Part print with two shaded views. Sizes in mm from the minimum x, y, z corner. Round coordinates to 2 decimals unless told otherwise and drop trailing zeros. Loops run counter-clockwise (first coordinate to the right, second up) from the corner with the lowest first, then second, coordinate; pieces in that order, holes last.
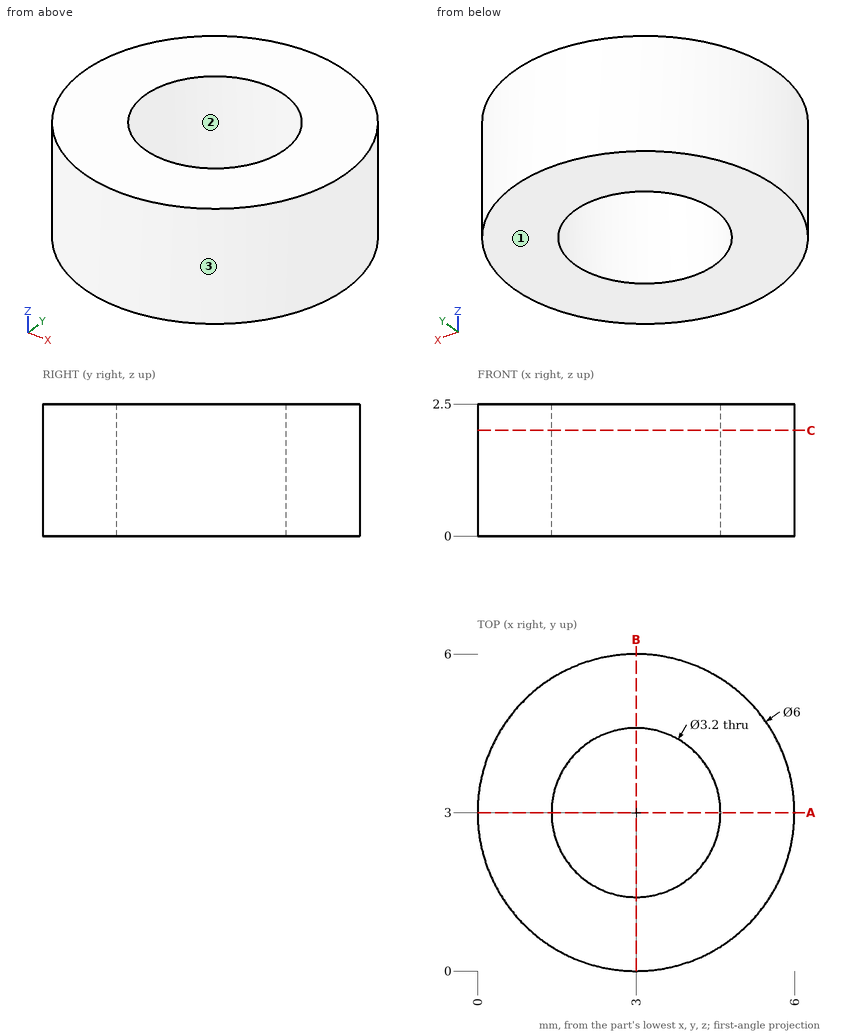
Item 1: Mould opens along Y. For the marked faces 1, 2 and 3 say: released by +Y, released by -Y, zero draft, split by the parting line, or undercut.
Verdict:
face 1: zero draft
face 2: undercut
face 3: split by the parting line
Item 2: Cut at A-A (y = 3). List the corners of the cut face in (x, z).
Verdict:
outline: (0, 0) - (1.4, 0) - (1.4, 2.5) - (0, 2.5) - close; (4.6, 0) - (6, 0) - (6, 2.5) - (4.6, 2.5) - close
Item 3: Cut at C-C (z = 2). List the corners of the cut face in (x, y), plus the area to 3 significant figures.
Verdict:
outline: circle Ø6 at (3, 3); hole circle Ø3.2 at (3, 3)
area: 20.2 mm2
Item 4: Wall check: L1, parallel to Y at x = 3, z = 1.3; L2, parallel to X at y = 3.15, z = 0.55; L3, parallel to Y at x = 4.2, z = 1.6. Give the ranges that are in metal, low to high.
Verdict:
L1: y = 0 to 1.4, 4.6 to 6
L2: x = 0 to 1.41, 4.59 to 6
L3: y = 0.25 to 1.94, 4.06 to 5.75
Item 5: Flat gauge pin, fed straight in: P1, Ø1, axis at x = 2, z = 2, coming from the -Y side. Where does the tip first touch, or does it go through?
Verdict:
P1: stops at y = 0.04
